For this review, take the finished solid that the model builds, in its own axes (mm). A direction names the side the tool comes from. Coordinates: 2 decimals unless noted, no trailing zeros. Order: outer loops, then holes, each group sorted by start corner. A loop starts at its lowest first (then second) coordinate and runs counter-clockwise, first axis right, second up. Notation, with made-up numbers: (22.5, 19.5) -> (44.5, 19.5) arc R27 cw to (44.5, 44.5) -> close; hole circle Ø8 at (19.25, 7). An arc over 180 degrees is marked (long way). Return JSON: item names as keys, results as strings. Group by question number.
Item 1: For line 1 along X through (y, z) = (1.45, -7); line 2 along Z through (x, y) = (-4.5, 0.8); line 3 along X through (y, z) = (-2.1, 46.5), list the stretches that pass through material, from the lowest coordinate up.
Item 2: Take a section at B-B (y = -1.75). Write out the cut boundary in (x, z).
Item 3: Draft analysis for pull direction X (two halves, no side actions). For faces 3 (the cylindrical face through (13.255, 0.986, -1.828)), 4 (the flat face through (-26.5, -1, 11)), 5 (the flat face through (42, -1, 11)), 6 (the flat face through (-25, -3, 26)), state which applies: +X half, -X half, draft (parallel to the pull), parting line (faces both ways), or undercut.
Item 4: Take a section at D-D (z = -28). Write out the cut boundary in (x, y), then the cut area to 3 significant figures.
Item 5: Machinability: for faces 1 (the flat face through (7, -1, 59.5)), 2 (the cylindrical face through (-0.58, 0.99, 37.04)), which of the approach directions +Z, -Z, +X, -X, +Y, -Y give a long, thin tool a straight path to every point of the face, cutting with its end or side? Answer none if there is none.
Item 6: Insertion check: pin 1 (10 mm diameter, centred on x = -4.5, z = 29.5, fed in from +Y). The pin has a flat end and moves straight along its axis. Give the tip position at first contact, or say it passes through.
Item 7: Take a section at A-A (x = 20). Write out the cut boundary in (y, z).
Item 8: Take a section at C-C (z = -7). Write out the cut boundary in (x, y).
```python
from build123d import *

# Parameters (mm, degrees)
CROQUIS1_W                   = 64.5
CROQUIS1_H                   = 96.5
CROQUIS1_R                   = 8.5
SALIENTE_EXTRUIR4_DEPTH      = 2
CROQUIS2_W                   = 68.5
CROQUIS2_H                   = 100.5
CROQUIS2_W_2                 = 64.5
CROQUIS2_H_2                 = 96.5
SALIENTE_EXTRUIR5_DEPTH      = 3
SALIENTE_EXTRUIR5_DEPTH_BACK = 2


with BuildPart() as part:
    # Croquis1 → Saliente-Extruir4 (new body)
    with BuildSketch(Plane(origin=(0, 0, 0), x_dir=(1, 0, 0), z_dir=(0, 1, 0))):
        with Locations((7.75, -11.25)):
            Rectangle(CROQUIS1_W, CROQUIS1_H)
        with Locations((20, -29.5)):
            Circle(CROQUIS1_R, mode=Mode.SUBTRACT)
        with Locations((-4.5, -29.5)):
            Circle(CROQUIS1_R, mode=Mode.SUBTRACT)
        with Locations((-4.5, 7)):
            Circle(CROQUIS1_R, mode=Mode.SUBTRACT)
        with Locations((20, 7)):
            Circle(CROQUIS1_R, mode=Mode.SUBTRACT)
    extrude(amount=SALIENTE_EXTRUIR4_DEPTH)

    # Croquis2 → Saliente-Extruir5 (add, two sides)
    with BuildSketch(Plane.XZ) as saliente_extruir5_sk:
        with Locations((7.75, 11.25)):
            Rectangle(CROQUIS2_W, CROQUIS2_H)
        with Locations((7.75, 11.25)):
            Rectangle(CROQUIS2_W_2, CROQUIS2_H_2, mode=Mode.SUBTRACT)
    extrude(amount=SALIENTE_EXTRUIR5_DEPTH)
    extrude(saliente_extruir5_sk.sketch, amount=-SALIENTE_EXTRUIR5_DEPTH_BACK)


solid = part.part
```
Findings below:
{
 "1": {"line 1": "x = -26.5 to -13, 4 to 11.5, 28.5 to 42", "line 2": "z = -39 to -15.5, 1.5 to 21, 38 to 61.5", "line 3": "x = -26.5 to -24.5, 40 to 42"},
 "2": {"outline": "(-26.5, -39) -> (42, -39) -> (42, 61.5) -> (-26.5, 61.5) -> close; hole (-24.5, -37) -> (40, -37) -> (40, 59.5) -> (-24.5, 59.5) -> close"},
 "3": {"face 3": "undercut", "face 4": "-X half", "face 5": "+X half", "face 6": "draft"},
 "4": {"outline": "(-26.5, -3) -> (-24.5, -3) -> (-24.5, 0) -> (40, 0) -> (40, -3) -> (42, -3) -> (42, 2) -> (-26.5, 2) -> close", "area": "149 mm2"},
 "5": {"face 1": "-Y", "face 2": "+Y, -Y"},
 "6": {"pin 1": "passes through"},
 "7": {"outline": "(-3, -39) -> (2, -39) -> (2, -15.5) -> (0, -15.5) -> (0, -37) -> (-3, -37) -> close; (-3, 59.5) -> (0, 59.5) -> (0, 38) -> (2, 38) -> (2, 61.5) -> (-3, 61.5) -> close; (0, 1.5) -> (2, 1.5) -> (2, 21) -> (0, 21) -> close"},
 "8": {"outline": "(-26.5, -3) -> (-24.5, -3) -> (-24.5, 0) -> (-13, 0) -> (-13, 2) -> (-26.5, 2) -> close; (4, 0) -> (11.5, 0) -> (11.5, 2) -> (4, 2) -> close; (28.5, 0) -> (40, 0) -> (40, -3) -> (42, -3) -> (42, 2) -> (28.5, 2) -> close"}
}
